Read the model definition and answer for the solid it produces. Units are mm, in the model's axes. Face numbers are marked on the shaded views. A direction names the side the tool comes from. Coordinates: 2 decimals unless noted, no trailing zeros. Order: outer loops, then holes, each group sorted by start corner. A loop starts at its lowest first (then second) coordinate and runs counter-clockwise, first axis right, second up. Notation, with made-up numbers: M -10,7 L 28,7 A23 cw 28,18 Z; hole C 17.25,-37.5 d6. An arc over 180 degrees is marked long. Put each result on its own line as item: value.
from build123d import *

# Parameters (mm, degrees)
MODEL_R                  = 4
RESSALTO_EXTRUS_O1_DEPTH = 6


with BuildPart() as part:
    # Model → Ressalto-extrusão1 (new body)
    with BuildSketch(Plane.XY):
        Polygon((52.38116631, 33.333915264), (57.481164074, 33.333915264), (57.481164074, 35.133913496), (64.481162154, 35.133913496), (64.481162154, 32.133915096), (64.413013807, 31.616277005), (64.213212962, 31.133915096), (63.895375717, 30.719701533), (63.481162154, 30.401864288), (62.998800244, 30.202063443), (62.481162154, 30.133915096), (58.481164074, 30.133915096), (58.481164074, 13.733926647), (52.981162794, 13.733926647), (52.981162794, 9.633928599), (52.913014447, 9.116290509), (52.713213602, 8.633928599), (52.395376357, 8.219715037), (51.981162794, 7.901877792), (51.498800885, 7.702076947), (50.981162794, 7.633928599), (47.981164394, 7.633928599), (47.981164394, 14.733926647), (49.781168706, 14.733926647), (49.781168706, 19.833924412), (41.781167571, 19.833924412), (41.781167571, 14.733926647), (43.581165802, 14.733926647), (43.581165802, 7.733928567), (40.581167402, 7.733928567), (40.063529312, 7.802076915), (39.581167402, 8.00187776), (39.16695384, 8.319715005), (38.849116595, 8.733928567), (38.64931575, 9.216290477), (38.581167402, 9.733928567), (38.581167402, 13.733926647), (29.081172202, 13.733926647), (29.081172202, 49.733913847), (42.081169322, 62.733910967), (58.481164074, 62.733910967), (58.481164074, 44.533910488), (62.581162122, 44.533910488), (63.098800212, 44.46576214), (63.581162122, 44.265961295), (63.995375685, 43.94812405), (64.31321293, 43.533910488), (64.513013775, 43.051548578), (64.581162122, 42.533910488), (64.581162122, 39.533912088), (57.481164074, 39.533912088), (57.481164074, 41.333916399), (52.38116631, 41.333916399), align=None)
        with Locations((38.95844444, 35.273938656)):
            Circle(MODEL_R, mode=Mode.SUBTRACT)
    extrude(amount=RESSALTO_EXTRUS_O1_DEPTH)


solid = part.part
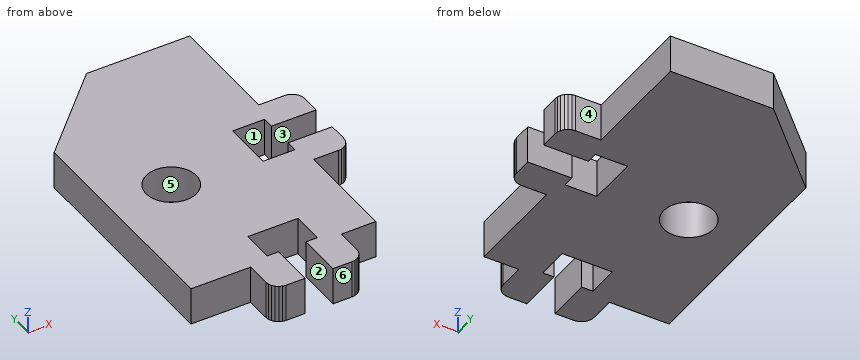
Q1. Find section A-A on y = 12. Write down the section's boundary in (x, z), plus the area to 3 significant figures.
Answers below:
outline: M 38.58,0 L 43.58,0 L 43.58,6 L 38.58,6 Z; M 47.98,0 L 52.98,0 L 52.98,6 L 47.98,6 Z
area: 60.0 mm^2
Q2. Consider line 1 along X through (y, z) = (40.5, 5.05); line 2 along X through (y, z) = (10, 1.35); line 3 along Y through (x, z) = (56.5, 0.9). Determine where each line is inside the solid, lowest interval first.
Answers below:
line 1: x = 29.08 to 52.38, 57.48 to 64.58
line 2: x = 38.58 to 43.58, 47.98 to 52.98
line 3: y = 13.73 to 33.33, 41.33 to 62.73
Q3. Find section B-B on x = 60. Write down the section's boundary in (y, z).
Answers below:
outline: M 30.13,0 L 35.13,0 L 35.13,6 L 30.13,6 Z; M 39.53,0 L 44.53,0 L 44.53,6 L 39.53,6 Z
Q4. Find section D-D on y = 28. Write down the section's boundary in (x, z).
Answers below:
outline: M 29.08,0 L 58.48,0 L 58.48,6 L 29.08,6 Z
Q5. A tool of negligible diameter and unlimited length cuts with its end or side. For the marked faces 1, 2 and 3, from which of +Z, -Z, +X, -X, +Y, -Y can it reach the whole face along a straight path? Write none if from no direction.
Answers below:
face 1: +Z, -Z
face 2: +Z, -Z, -Y
face 3: +Z, -Z, +X
Q6. For a pull along Y with two mould halves and no side action, classify the marked faces 4, 5 and 6 as +Y half, -Y half, draft (parallel to the pull), parting line (faces both ways), or undercut.
Answers below:
face 4: +Y half
face 5: undercut
face 6: -Y half
Q7. Given pin 1 (3 mm diameter, centred on x = 37.5, z = 5, fed in from -Y); pin 2 (3 mm diameter, centred on x = 61.5, z = 4, fed in from -Y); pin 3 (1 mm diameter, centred on y = 55, z = 5, fed in from +X), each flat-ended and moving along its own axis, determine where each tip first touches the part or whether it passes through.
Answers below:
pin 1: stops at y = 8.54
pin 2: stops at y = 30.13
pin 3: stops at x = 58.48
Q8. Find section C-C on x = 47. Write down the section's boundary in (y, z), plus the area to 3 significant figures.
Answers below:
outline: M 19.83,0 L 62.73,0 L 62.73,6 L 19.83,6 Z
area: 257 mm^2
